Part model, mm, in its own coordinate system. Face numbers are marked on the shaded views. Give positions to 0.01 mm unless a question says otherwise; leave off trailing zeros. Write each loop counter-clockwise with the first axis right and the second up, starting at its lowest first coordinate (ties: lowest second). Pieces come first, ordered by that corner, then holes. Notation, with made-up numbers: (-35.75, 32) - (-8.75, 32) arc R20 ccw to (-8.75, 43) - close; hole circle Ø9 at (-15, -7). An arc over 180 degrees is marked (long way). Answer as a JSON object with one key per item and string values. Group by question number.
Autodesk Inventor part; units mm, degrees
ref_plane "YZ Plane" through (0, 0, 0) normal (1, 0, 0) x (0, 1, 0)
ref_plane "XZ Plane" through (0, 0, 0) normal (0, 1, 0) x (-1, 0, 0)
ref_plane "XY Plane" through (0, 0, 0) normal (0, 0, 1) x (1, 0, 0)
sketch "Sketch1" plane through (0, 0, 0) normal (0, 1, 0) x (-1, 0, 0)
  circle A0 centre (0, 0) radius 4
  circle A1 centre (0, 0) radius 7
  dimension "d0" = 8
  dimension "d1" = 14
extrude "Extrusion1" add sketch "Sketch1" along normal blind 25
chamfer "Chamfer1" distance 1 angle 45 4 edges at (7, 25, 0) (7, 0, 0) (4, 25, 0) (4, 0, 0)
sketch "Sketch2" plane through (0, 0, 0) normal (1, 0, 0) x (0, 1, 0)
  circle A0 centre (20, 0) radius 1.6
  circle A1 centre (5, 0) radius 1.6
  line L0 (0, 0) -> (25, 0)
  line L1 (25, 6) -> (25, -6)
  line L2 (0, -6) -> (0, 6)
  dimension "d7" = 3.2
  dimension "d8" = 3.2
  dimension "d9" = 5
  dimension "d10" = 5
extrude "Extrusion2" cut sketch "Sketch2" along normal mid plane 25
properties part number "Acople"
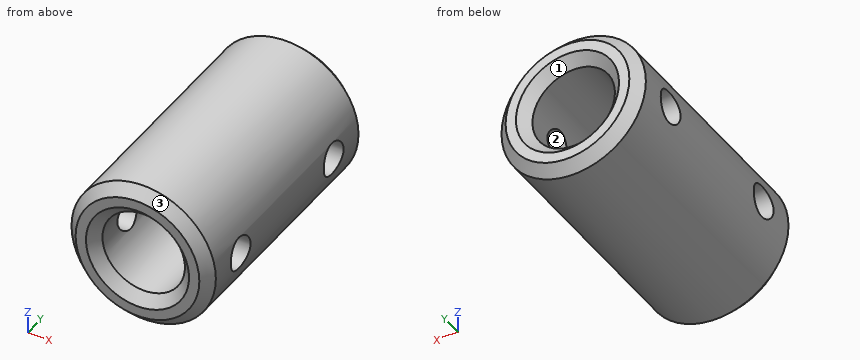
1) Band-saw the part on B-B (x = 0). List the corners of the cut face in (y, z), plus the area to 3 significant figures.
2) Mould opens along X. For the marked faces 1, 2 and 3 say: pulls with the +X half, pulls with the -X half, needs draft (parallel to the pull), parting line crosses it, or undercut.
3) Drop flat-ended pins along their axis: P1, Ø1.5, axis at y = 22.5, z = 1.5, coming from the -X side; P2, Ø1, axis at x = -1.5, z = 0.5, coming from the -Y side; P3, Ø3, axis at y = 15.5, z = 2.5, coming from the +X side; P4, Ø1, axis at y = 16.5, z = 5.5, coming from the +X side. Give the stop position or say it passes through.
4) Band-saw the part on A-A (z = 0). State how many separate pieces and enclosed holes the cut face has, plus the area to 3 significant figures.
5) Probe line 1 (Z direction, x = 0, y = 12.5); line 2 (Z direction, x = -5, y = 20). List the from-to ranges inside material, lowest first.
6) Band-saw the part on D-D (y = 10). List the corners of the cut face in (x, z).
7) Band-saw the part on C-C (y = 4.5). List the corners of the cut face in (x, z).
Verdict:
{
 "1": {"outline": "(0, -6) - (1, -7) - (24, -7) - (25, -6) - (25, -5) - (24, -4) - (1, -4) - (0, -5) - close; (0, 5) - (1, 4) - (24, 4) - (25, 5) - (25, 6) - (24, 7) - (1, 7) - (0, 6) - close", "area": "146 mm2"},
 "2": {"face 1": "undercut", "face 2": "needs draft", "face 3": "parting line crosses it"},
 "3": {"P1": "x = -6.96", "P2": "through", "P3": "x = 6.93", "P4": "x = 4.9"},
 "4": {"separate pieces": "6", "enclosed holes": "0", "area": "108 mm2"},
 "5": {"line 1": "-7 to -4, 4 to 7", "line 2": "-4.9 to -1.6, 1.6 to 4.9"},
 "6": {"outline": "circle Ø14 at (0, 0); hole circle Ø8 at (0, 0)"},
 "7": {"outline": "(-6.83, -1.52) arc R7 ccw to (6.83, -1.52) - (3.7, -1.52) arc R4 cw to (-3.7, -1.52) - close; (-6.83, 1.52) - (-3.7, 1.52) arc R4 cw to (3.7, 1.52) - (6.83, 1.52) arc R7 ccw to start"}
}
